Read the model definition and answer for the solid it produces. Units are mm, in the model's axes. Give positions to 0.01 mm unless a question says otherwise; leave off trailing zeros. Write each loop counter-clockwise with the first axis right and the second up, starting at its lowest first coordinate (ties: lowest second). Pieces come first, ordered by that corner, then holes. Notation, with made-up numbers: M 16.5,-35.5 L 67.5,-35.5 A21 cw 67.5,-31.5 Z; hole C 38,15 d9. An arc over 180 degrees is marked long. Put each result on its own line as item: value.
Autodesk Inventor part; units mm, degrees
ref_plane "YZ Plane" through (0, 0, 0) normal (1, 0, 0) x (0, 1, 0)
ref_plane "XZ Plane" through (0, 0, 0) normal (0, 1, 0) x (-1, 0, 0)
ref_plane "XY Plane" through (0, 0, 0) normal (0, 0, 1) x (1, 0, 0)
sketch "Sketch1" plane through (0, 0, 0) normal (0, 1, 0) x (-1, 0, 0)
  line L0 (50, 25) -> (-50, 25)
  line L1 (-50, 25) -> (-50, -25)
  line L2 (-50, -25) -> (50, -25)
  line L3 (50, -25) -> (50, 25)
  line L4 (50, 25) -> (-50, -25) construction
  line L5 (-50, 25) -> (50, -25) construction
  point P0 (0, 0)
  dimension "d0" = 100
  dimension "d1" = 50
extrude "Extrusion1" add sketch "Sketch1" along normal blind 6
fillet "Fillet1" radius 5 4 edges at (50, 3, 25) (50, 3, -25) (-50, 3, -25) (-50, 3, 25)
sketch "Sketch2" plane through (0, 6, 0) normal (0, 1, 0) x (1, 0, 0)
  line L0 (-39.5, -21.25) -> (-30.5, -21.25)
  line L1 (-30.5, -21.25) -> (-30.5, -4.75)
  line L2 (-30.5, -4.75) -> (-39.5, -4.75)
  line L3 (-39.5, -4.75) -> (-39.5, -21.25)
  line L4 (-39.5, -21.25) -> (-30.5, -4.75) construction
  line L5 (-30.5, -21.25) -> (-39.5, -4.75) construction
  line L6 (-25.5, -21.25) -> (-16.5, -21.25)
  line L7 (-16.5, -21.25) -> (-16.5, -4.75)
  line L8 (-16.5, -4.75) -> (-25.5, -4.75)
  line L9 (-25.5, -4.75) -> (-25.5, -21.25)
  line L10 (-25.5, -21.25) -> (-16.5, -4.75) construction
  line L11 (-16.5, -21.25) -> (-25.5, -4.75) construction
  line L12 (-11.5, -21.25) -> (-2.5, -21.25)
  line L13 (-2.5, -21.25) -> (-2.5, -4.75)
  line L14 (-2.5, -4.75) -> (-11.5, -4.75)
  line L15 (-11.5, -4.75) -> (-11.5, -21.25)
  line L16 (-11.5, -21.25) -> (-2.5, -4.75) construction
  line L17 (-2.5, -21.25) -> (-11.5, -4.75) construction
  line L18 (2.5, -21.25) -> (11.5, -21.25)
  line L19 (11.5, -21.25) -> (11.5, -4.75)
  line L20 (11.5, -4.75) -> (2.5, -4.75)
  line L21 (2.5, -4.75) -> (2.5, -21.25)
  line L22 (2.5, -21.25) -> (11.5, -4.75) construction
  line L23 (11.5, -21.25) -> (2.5, -4.75) construction
  line L24 (16.5, -21.25) -> (25.5, -21.25)
  line L25 (25.5, -21.25) -> (25.5, -4.75)
  line L26 (25.5, -4.75) -> (16.5, -4.75)
  line L27 (16.5, -4.75) -> (16.5, -21.25)
  line L28 (16.5, -21.25) -> (25.5, -4.75) construction
  line L29 (25.5, -21.25) -> (16.5, -4.75) construction
  line L30 (30.5, -21.25) -> (39.5, -21.25)
  line L31 (39.5, -21.25) -> (39.5, -4.75)
  line L32 (39.5, -4.75) -> (30.5, -4.75)
  line L33 (30.5, -4.75) -> (30.5, -21.25)
  line L34 (30.5, -21.25) -> (39.5, -4.75) construction
  line L35 (39.5, -21.25) -> (30.5, -4.75) construction
  point P0 (0, 0)
  point P1 (-35, -13)
  point P2 (-21, -13)
  point P3 (-7, -13)
  point P4 (7, -13)
  point P5 (21, -13)
  point P6 (35, -13)
  dimension "d5" = 9
  dimension "d6" = 16.5
  dimension "d9" = 14
  dimension "d14" = 7
  dimension "d15" = 13
extrude "Extrusion2" cut sketch "Sketch2" against normal blind 10
sketch "Sketch3" plane through (0, 6, 0) normal (0, 1, 0) x (1, 0, 0)
  line L0 (-16.5, -21.25) -> (-25.5, -21.25)
  line L1 (-45, -25) -> (45, -25)
  line L2 (45, 25) -> (-45, 25)
  line L3 (-38, 0) -> (-32, 0)
  line L4 (-32, 0) -> (-32, 20)
  line L5 (-32, 20) -> (-38, 20)
  line L6 (-38, 20) -> (-38, 0)
  line L7 (-38, 0) -> (-32, 20) construction
  line L8 (-32, 0) -> (-38, 20) construction
  line L9 (-24, 0) -> (-18, 0)
  line L10 (-18, 0) -> (-18, 20)
  line L11 (-18, 20) -> (-24, 20)
  line L12 (-24, 20) -> (-24, 0)
  line L13 (-24, 0) -> (-18, 20) construction
  line L14 (-18, 0) -> (-24, 20) construction
  line L15 (-10, 0) -> (-4, 0)
  line L16 (-4, 0) -> (-4, 20)
  line L17 (-4, 20) -> (-10, 20)
  line L18 (-10, 20) -> (-10, 0)
  line L19 (-10, 0) -> (-4, 20) construction
  line L20 (-4, 0) -> (-10, 20) construction
  line L21 (4, 0) -> (10, 0)
  line L22 (10, 0) -> (10, 20)
  line L23 (10, 20) -> (4, 20)
  line L24 (4, 20) -> (4, 0)
  line L25 (4, 0) -> (10, 20) construction
  line L26 (10, 0) -> (4, 20) construction
  line L27 (18, 0) -> (24, 0)
  line L28 (24, 0) -> (24, 20)
  line L29 (24, 20) -> (18, 20)
  line L30 (18, 20) -> (18, 0)
  line L31 (18, 0) -> (24, 20) construction
  line L32 (24, 0) -> (18, 20) construction
  line L33 (32, 0) -> (38, 0)
  line L34 (38, 0) -> (38, 20)
  line L35 (38, 20) -> (32, 20)
  line L36 (32, 20) -> (32, 0)
  line L37 (32, 0) -> (38, 20) construction
  line L38 (38, 0) -> (32, 20) construction
  point P0 (0, 0)
  point P1 (-35, 10)
  point P2 (-21, 10)
  point P3 (-7, 10)
  point P4 (7, 10)
  point P5 (21, 10)
  point P6 (35, 10)
  dimension "d20" = 14
  dimension "d25" = 7
  dimension "d26" = 6
  dimension "d27" = 20
  dimension "d28" = 5
  dimension "d29" = 3.75
extrude "Extrusion3" cut sketch "Sketch3" against normal blind 10
sketch "Sketch4" plane through (0, 6, 0) normal (0, 1, 0) x (1, 0, 0)
  arc A0 (-50, -20) -> (-45, -25) centre (-45, -20) ccw
  arc A1 (45, -25) -> (50, -20) centre (45, -20) ccw
  arc A2 (50, 20) -> (45, 25) centre (45, 20) ccw
  arc A3 (-45, 25) -> (-50, 20) centre (-45, 20) ccw
  point P0 (0, 0)
hole "Hole1" at (-45, 6, -20) at (45, 6, -20) at (45, 6, 20) at (-45, 6, 20) direction (0, -1, 0) diameter 4 end through all
sketch "Sketch5" plane through (0, 6, 0) normal (0, 1, 0) x (1, 0, 0)
  line L0 (-30.5, -4.75) -> (-30.5, -21.25)
  line L1 (-39.5, -4.75) -> (-30.5, -4.75)
  line L2 (-25.5, -21.25) -> (-25.5, -4.75)
  line L3 (-25.5, -16.5) -> (-30.5, -16.5)
  line L4 (-30.5, -16.5) -> (-30.5, -9.5)
  line L5 (-30.5, -9.5) -> (-25.5, -9.5)
  line L6 (-25.5, -9.5) -> (-25.5, -16.5)
  line L7 (-25.5, -16.5) -> (-30.5, -9.5) construction
  line L8 (-30.5, -16.5) -> (-25.5, -9.5) construction
  line L9 (-11.5, -16.5) -> (-16.5, -16.5)
  line L10 (-16.5, -16.5) -> (-16.5, -9.5)
  line L11 (-16.5, -9.5) -> (-11.5, -9.5)
  line L12 (-11.5, -9.5) -> (-11.5, -16.5)
  line L13 (-11.5, -16.5) -> (-16.5, -9.5) construction
  line L14 (-16.5, -16.5) -> (-11.5, -9.5) construction
  line L15 (2.5, -16.5) -> (-2.5, -16.5)
  line L16 (-2.5, -16.5) -> (-2.5, -9.5)
  line L17 (-2.5, -9.5) -> (2.5, -9.5)
  line L18 (2.5, -9.5) -> (2.5, -16.5)
  line L19 (2.5, -16.5) -> (-2.5, -9.5) construction
  line L20 (-2.5, -16.5) -> (2.5, -9.5) construction
  line L21 (16.5, -16.5) -> (11.5, -16.5)
  line L22 (11.5, -16.5) -> (11.5, -9.5)
  line L23 (11.5, -9.5) -> (16.5, -9.5)
  line L24 (16.5, -9.5) -> (16.5, -16.5)
  line L25 (16.5, -16.5) -> (11.5, -9.5) construction
  line L26 (11.5, -16.5) -> (16.5, -9.5) construction
  line L27 (30.5, -16.5) -> (25.5, -16.5)
  line L28 (25.5, -16.5) -> (25.5, -9.5)
  line L29 (25.5, -9.5) -> (30.5, -9.5)
  line L30 (30.5, -9.5) -> (30.5, -16.5)
  line L31 (30.5, -16.5) -> (25.5, -9.5) construction
  line L32 (25.5, -16.5) -> (30.5, -9.5) construction
  line L33 (44.5, -16.5) -> (39.5, -16.5)
  line L34 (39.5, -16.5) -> (39.5, -9.5)
  line L35 (39.5, -9.5) -> (44.5, -9.5)
  line L36 (44.5, -9.5) -> (44.5, -16.5)
  line L37 (44.5, -16.5) -> (39.5, -9.5) construction
  line L38 (39.5, -16.5) -> (44.5, -9.5) construction
  point P0 (-39.5, -21.25)
  point P1 (0, 0)
  point P2 (-28, -13)
  point P3 (-14, -13)
  point P4 (0, -13)
  point P5 (14, -13)
  point P6 (28, -13)
  point P7 (42, -13)
  dimension "d39" = 0
  dimension "d40" = 7
  dimension "d41" = 16.5
  dimension "d42" = 8.25
  dimension "d45" = 14
extrude "Extrusion4" cut sketch "Sketch5" against normal blind 10
sketch "Sketch6" plane through (0, 6, 0) normal (0, 1, 0) x (1, 0, 0)
  line L0 (-32, 20) -> (-32, 0)
  line L1 (-32, 0) -> (-38, 0)
  line L2 (-38, 20) -> (-32, 20)
  line L3 (-26, -3) -> (-32, -3)
  line L4 (-32, -3) -> (-32, 13)
  line L5 (-32, 13) -> (-26, 13)
  line L6 (-26, 13) -> (-26, -3)
  line L7 (-26, -3) -> (-32, 13) construction
  line L8 (-32, -3) -> (-26, 13) construction
  line L9 (-12, -3) -> (-18, -3)
  line L10 (-18, -3) -> (-18, 13)
  line L11 (-18, 13) -> (-12, 13)
  line L12 (-12, 13) -> (-12, -3)
  line L13 (-12, -3) -> (-18, 13) construction
  line L14 (-18, -3) -> (-12, 13) construction
  line L15 (2, -3) -> (-4, -3)
  line L16 (-4, -3) -> (-4, 13)
  line L17 (-4, 13) -> (2, 13)
  line L18 (2, 13) -> (2, -3)
  line L19 (2, -3) -> (-4, 13) construction
  line L20 (-4, -3) -> (2, 13) construction
  line L21 (16, -3) -> (10, -3)
  line L22 (10, -3) -> (10, 13)
  line L23 (10, 13) -> (16, 13)
  line L24 (16, 13) -> (16, -3)
  line L25 (16, -3) -> (10, 13) construction
  line L26 (10, -3) -> (16, 13) construction
  line L27 (30, -3) -> (24, -3)
  line L28 (24, -3) -> (24, 13)
  line L29 (24, 13) -> (30, 13)
  line L30 (30, 13) -> (30, -3)
  line L31 (30, -3) -> (24, 13) construction
  line L32 (24, -3) -> (30, 13) construction
  line L33 (44, -3) -> (38, -3)
  line L34 (38, -3) -> (38, 13)
  line L35 (38, 13) -> (44, 13)
  line L36 (44, 13) -> (44, -3)
  line L37 (44, -3) -> (38, 13) construction
  line L38 (38, -3) -> (44, 13) construction
  point P0 (0, 0)
  point P1 (-29, 5)
  point P2 (-18, 0)
  point P3 (-15, 5)
  point P4 (-4, 0)
  point P5 (-1, 5)
  point P6 (10, 0)
  point P7 (13, 5)
  point P8 (24, 0)
  point P9 (27, 5)
  point P10 (38, 0)
  point P11 (41, 5)
  dimension "d52" = 6
  dimension "d53" = 3
  dimension "d54" = 7
  dimension "d57" = 14
extrude "Extrusion5" cut sketch "Sketch6" against normal blind 10
properties part number "AcrylicUpperCore" material "Acrylic, Clear"
(1) Section B-B on x = 27.5 is taken. Determine the outline of the cut face in (y, z).
Result:
outline: M 0,-25 L 6,-25 L 6,-13 L 0,-13 Z; M 0,3 L 6,3 L 6,9.5 L 0,9.5 Z; M 0,16.5 L 6,16.5 L 6,25 L 0,25 Z
(2) Section C-C on z = 15 is taken. Determine the outline of the cut face in (x, y), and give its area (3 significant figures).
Result:
outline: M -50,0 L -39.5,0 L -39.5,6 L -50,6 Z; M 44.5,0 L 50,0 L 50,6 L 44.5,6 Z
area: 96.0 mm²
(3) Section D-D on y = 3.7 is taken. Give the number of separate pieces and of enclosed holes in the cut face, and give its area (3 significant figures).
Result:
separate pieces: 1
enclosed holes: 11
area: 2,530 mm²
(4) For a pull along Z with two mould halves and no side action, classify faces 1 (the face through (25.5, 3, 7)), 2 (the face through (49, 3, -23)) as +Z half, -Z half, draft (parallel to the pull), parting line (faces both ways), or undercut.
Result:
face 1: undercut
face 2: -Z half
(5) Section A-A on z = -2 is taken. Determine the outline of the cut face in (x, y), and give its area (3 significant figures).
Result:
outline: M -50,0 L -38,0 L -38,6 L -50,6 Z; M -26,0 L -24,0 L -24,6 L -26,6 Z; M -12,0 L -10,0 L -10,6 L -12,6 Z; M 2,0 L 4,0 L 4,6 L 2,6 Z; M 16,0 L 18,0 L 18,6 L 16,6 Z; M 30,0 L 32,0 L 32,6 L 30,6 Z; M 44,0 L 50,0 L 50,6 L 44,6 Z
area: 168 mm²
(6) Given pin 1 Ø6 at (x, z) = (35, 12.5) entering from -Y, flat-ended and moving along its own axis, determine where the tip first touches the part or whether it passes through.
Result:
pin 1: passes through
(7) Straight lines are drawn through the part: line 1 along Z through (x, y) = (21.5, 4.7); line 2 along Z through (x, y) = (40, 5); line 3 along X through (y, z) = (2.5, 14). For each, find the intervals that lie inside material, in ascending order. Write a range as from..to.
Result:
line 1: z = -25..-20, 0..4.75, 21.25..25
line 2: z = -25..-13, 3..9.5, 16.5..25
line 3: x = -50..-39.5, 44.5..50
